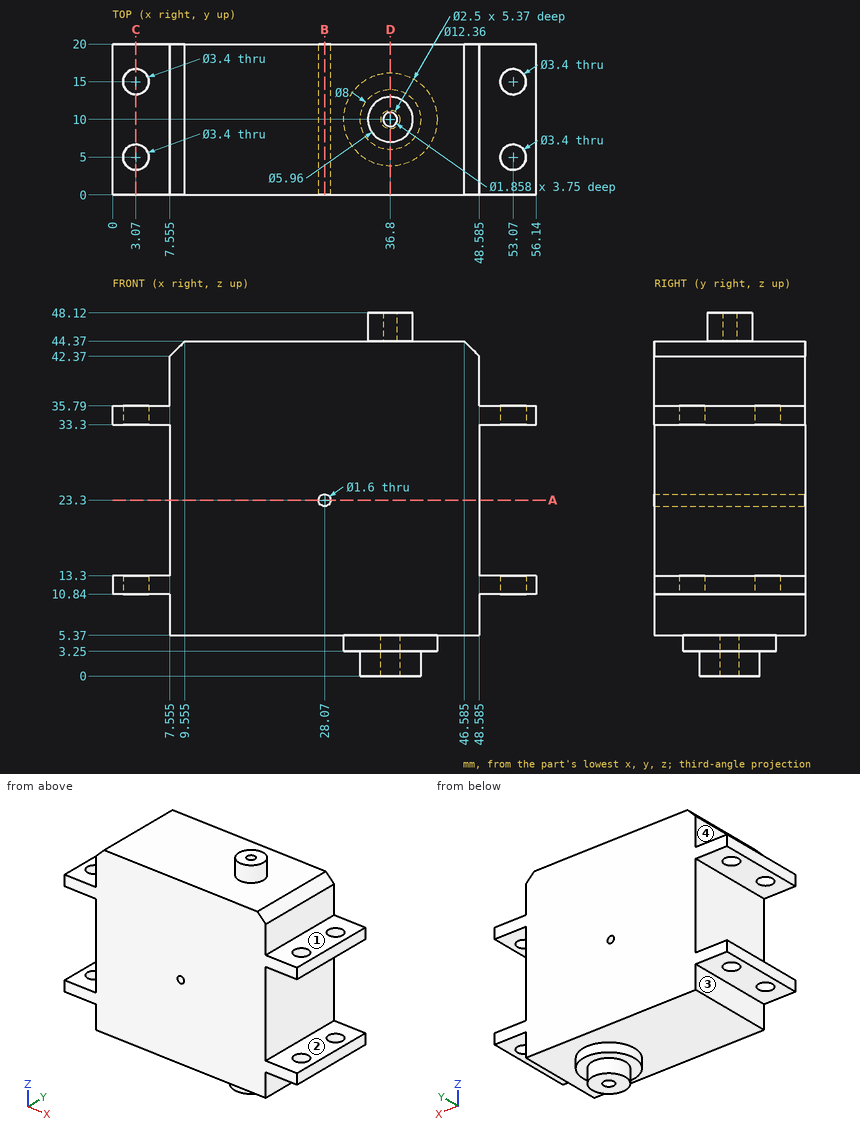
Input: dimensioned drawing with shaded views. Units: mm. Origin: part minimum x, y, z. A direction names the side the tool comes from. Coordinates: 2 decimals unless noted, no trailing zeros. Order: outer loops, then holes, each group sorted by start corner. A loop starts at its lowest first (then second) coordinate and runs counter-clockwise, first axis right, second up. Notation, with made-up numbers: (65, -10) - (117, -10) arc R24 cw to (117, 20) - close; hole circle Ø6 at (69, 36.5). An arc over 180 degrees is marked (long way). Return JSON: item names as keys, results as strings. Group by question number.
1. Cut plane D-D (x = 36.8). Output: boundary loops of the cut face in (y, z), plus the area to 3 significant figures.
2. Pin query (flat end, axial travel): pin 1 (12 mm diameter, centred on x = 19.5, z = 12, fed in from -Y); pin 2 (2.5 mm diameter, centred on x = 51.5, y = 6.5, fed in from +Z); pin 3 (6 mm diameter, centred on x = 24, y = 11.5, fed in from +Z); pin 4 (8.5 mm diameter, centred on x = 51.5, y = 6.5, fed in from -Z). Return the tip coordinate at first contact, or that it passes through.
3. Cut plane C-C (x = 3.07). Output: boundary loops of the cut face in (y, z).
4. Material intervals for line 1 along X through (y, z) = (5, 12.25); line 2 along Y through (x, z) = (53.07, 34.25); line 3 along X through (y, z) = (14.5, 23.3) (3 decimals), sorted ascending. Write a range as [from, to].
5. Set-up query: the marked faces 1, 2, 3 and 4. Return all of +Z, -Z, +X, -X, +Y, -Y with unobstructed straight access to the full face (end or side cutting, diameter ignored); none if empty.
6. Cut plane B-B (x = 28.07). Output: boundary loops of the cut face in (y, z), plus the area to 3 significant figures.
7. Cut plane A-A (z = 23.3). Output: boundary loops of the cut face in (x, y) (3 decimals).
Resolved:
{
 "1": {"outline": "(0, 5.37) - (3.82, 5.37) - (3.82, 3.25) - (6, 3.25) - (6, 0) - (8.75, 0) - (8.75, 5.37) - (11.25, 5.37) - (11.25, 0) - (14, 0) - (14, 3.25) - (16.18, 3.25) - (16.18, 5.37) - (20, 5.37) - (20, 44.37) - (12.98, 44.37) - (12.98, 48.12) - (10.93, 48.12) - (10.93, 44.37) - (9.07, 44.37) - (9.07, 48.12) - (7.02, 48.12) - (7.02, 44.37) - (0, 44.37) - close", "area": "834 mm²"},
 "2": {"pin 1": "stops at y = 0", "pin 2": "stops at z = 35.79", "pin 3": "stops at z = 44.37", "pin 4": "stops at z = 5.37"},
 "3": {"outline": "(0, 10.84) - (3.3, 10.84) - (3.3, 13.3) - (0, 13.3) - close; (0, 33.3) - (3.3, 33.3) - (3.3, 35.79) - (0, 35.79) - close; (6.7, 10.84) - (13.3, 10.84) - (13.3, 13.3) - (6.7, 13.3) - close; (6.7, 33.3) - (13.3, 33.3) - (13.3, 35.79) - (6.7, 35.79) - close; (16.7, 10.84) - (20, 10.84) - (20, 13.3) - (16.7, 13.3) - close; (16.7, 33.3) - (20, 33.3) - (20, 35.79) - (16.7, 35.79) - close"},
 "4": {"line 1": "x = [0, 1.37], [4.77, 51.37], [54.77, 56.14]", "line 2": "y = [0, 3.3], [6.7, 13.3], [16.7, 20]", "line 3": "x = [7.555, 27.27], [28.87, 48.585]"},
 "5": {"face 1": "+Z, +X, +Y, -Y", "face 2": "+X, +Y, -Y", "face 3": "-Z, -X, +Y, -Y", "face 4": "+Z, -X, +Y, -Y"},
 "6": {"outline": "(0, 5.37) - (20, 5.37) - (20, 22.5) - (0, 22.5) - close; (0, 24.1) - (20, 24.1) - (20, 44.37) - (0, 44.37) - close", "area": "748 mm²"},
 "7": {"outline": "(7.555, 0) - (27.27, 0) - (27.27, 20) - (7.555, 20) - close; (28.87, 0) - (48.585, 0) - (48.585, 20) - (28.87, 20) - close"}
}
